The listing builds one solid part. Answer for the finished solid, in the listing's coordinates (mm). Round coordinates to 2 decimals unless told otherwise and drop trailing zeros. Write each loop counter-clockwise with the first axis right and the second up, starting at its lowest first coordinate (ties: lowest second). Pieces come first, ordered by that corner, then holes. Notation, with made-up numbers: M 88,30.25 L 135,30.25 A13 cw 135,38.25 Z; hole C -6,51.25 d7. An arc over 180 degrees is marked long. Write each question's results on one line, items separated by ' | '.
from build123d import *

# Parameters (mm, degrees)
SKETCH1_W           = 30
SKETCH1_H           = 25
SKETCH1_R           = 7.5
BOSS_EXTRUDE1_DEPTH = 18
SKETCH3_R           = 2
CUT_EXTRUDE1_DEPTH  = 35.263683398


with BuildPart() as part:
    # Sketch1 → Boss-Extrude1 (new body)
    with BuildSketch(Plane.XY):
        Rectangle(SKETCH1_W, SKETCH1_H)
        Circle(SKETCH1_R, mode=Mode.SUBTRACT)
    extrude(amount=BOSS_EXTRUDE1_DEPTH)

    # Sketch3 → Cut-Extrude1 (cut, through all)
    with BuildSketch(Plane(origin=(0, 12.5, 0), x_dir=(1, 0, 0), z_dir=(0, 1, 0))):
        with Locations(Location((-10, -9, 0), (0, 0, 270))):
            Circle(SKETCH3_R)
        with Locations(Location((10, -9, 0), (0, 0, 90))):
            Circle(SKETCH3_R)
    extrude(amount=-CUT_EXTRUDE1_DEPTH, mode=Mode.SUBTRACT)


solid = part.part
1) Section D-D (z = 6.5) is taken. Determine the outline of the cut face in (x, y).
Return value:
outline: M -15,-12.5 L 15,-12.5 L 15,12.5 L -15,12.5 Z; hole C 0,0 d15
2) Section A-A (z = 9) is taken. Determine the outline of the cut face in (x, y).
Return value:
outline: M -15,-12.5 L -12,-12.5 L -12,12.5 L -15,12.5 Z; M -8,-12.5 L 8,-12.5 L 8,12.5 L -8,12.5 Z; M 12,-12.5 L 15,-12.5 L 15,12.5 L 12,12.5 Z; hole C 0,0 d15
3) Section B-B (x = 10) is taken. Determine the outline of the cut face in (y, z), then the cut area to 3 significant figures.
Return value:
outline: M -12.5,0 L 12.5,0 L 12.5,7 L -12.5,7 Z; M -12.5,11 L 12.5,11 L 12.5,18 L -12.5,18 Z | area: 350 mm²
4) Each of these flat-tipped pins is pushed along its axis until it touches: pin 1 (10 mm diameter, centred on x = -9.5, z = 8.5, fed in from -Y); pin 2 (3.5 mm diameter, centred on x = 10, z = 9, fed in from +Y). Where does it stop, or does it pass through?
Return value:
pin 1: y = -12.5 | pin 2: through
5) Find the intervals of material crossed by line 1 (Z direction, x = 10, y = -0.5); line 2 (Y direction, x = 0, z = 5.5); line 3 (X direction, y = -8, z = 8.5), in increasing order.
Return value:
line 1: 0 to 7, 11 to 18 | line 2: -12.5 to -7.5, 7.5 to 12.5 | line 3: -15 to -11.94, -8.06 to 8.06, 11.94 to 15
6) The mould has two halves that part along Y. Classify faces 1 (the face through (-7.493, 0.33, 8.874)), 2 (the face through (0, 9, 18)), 3 (the face through (0, -12.5, 9)): +Y half, -Y half, draft (parallel to the pull), parting line (faces both ways), or undercut.
Return value:
face 1: undercut | face 2: draft | face 3: -Y half
7) Section C-C (y = 0) is taken. Determine the outline of the cut face in (x, z), then the cut area to 3 significant figures.
Return value:
outline: M -15,0 L -7.5,0 L -7.5,18 L -15,18 Z; M 7.5,0 L 15,0 L 15,18 L 7.5,18 Z; hole C -10,9 d4; hole C 10,9 d4 | area: 245 mm²
